from build123d import *

# Parameters (mm, degrees)
SKETCH1_W           = 80
SKETCH1_H           = 100
SKETCH1_R           = 2.1
SKETCH1_R_2         = 2.5
BOSS_EXTRUDE1_DEPTH = 3


with BuildPart() as part:
    # Sketch1 → Boss-Extrude1 (new body)
    with BuildSketch(Plane(origin=(0, 0, 0), x_dir=(1, 0, 0), z_dir=(0, 1, 0))):
        Rectangle(SKETCH1_W, SKETCH1_H)
        with Locations(Location((24.5, 42, 0), (0, 0, 90))):
            Circle(SKETCH1_R, mode=Mode.SUBTRACT)
        with Locations(Location((-24.5, 42, 0), (0, 0, 270))):
            Circle(SKETCH1_R, mode=Mode.SUBTRACT)
        with Locations(Location((24.5, -40, 0), (0, 0, 270))):
            Circle(SKETCH1_R, mode=Mode.SUBTRACT)
        with Locations(Location((-24.5, -40, 0), (0, 0, 270))):
            Circle(SKETCH1_R, mode=Mode.SUBTRACT)
        with Locations(Location((10, -10, 0), (0, 0, 270))):
            Circle(SKETCH1_R, mode=Mode.SUBTRACT)
        with Locations(Location((-10, -10, 0), (0, 0, 270))):
            Circle(SKETCH1_R, mode=Mode.SUBTRACT)
        with Locations(Location((0, -27, 0), (0, 0, 270))):
            Circle(SKETCH1_R_2, mode=Mode.SUBTRACT)
    extrude(amount=BOSS_EXTRUDE1_DEPTH)


solid = part.part
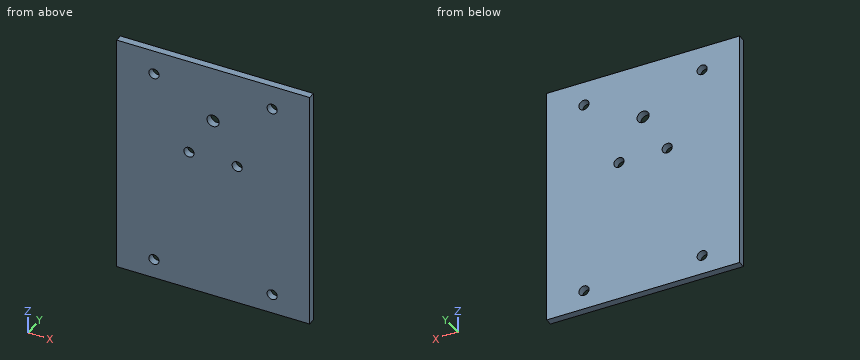
Source: CAD feature listing. Evaluate the final solid. Frame: model axes, mm. Give positions to 0.01 mm unless a question says otherwise; leave off trailing zeros. Write each loop counter-clockwise with the first axis right and the second up, starting at its lowest first coordinate (ties: lowest second). Pieces come first, ordered by that corner, then holes. Notation, with made-up numbers: M 53,67 L 67,67 A16 cw 67,73 Z; hole C 40,-13 d10. An arc over 180 degrees is marked long. Answer as a JSON object with one key per item and string values.
Q1. Cut plane C-C, the plane x = 24.5. Return the cut outline in (y, z).
Geometry check:
{"outline": "M 0,-50 L 3,-50 L 3,-44.1 L 0,-44.1 Z; M 0,-39.9 L 3,-39.9 L 3,37.9 L 0,37.9 Z; M 0,42.1 L 3,42.1 L 3,50 L 0,50 Z"}
Q2. Cut plane B-B, the plane x = 0. Return the cut outline in (y, z), then the cut area to 3 significant figures.
Geometry check:
{"outline": "M 0,-50 L 3,-50 L 3,24.5 L 0,24.5 Z; M 0,29.5 L 3,29.5 L 3,50 L 0,50 Z", "area": "285 mm^2"}
Q3. Cut plane A-A, the plane z = 27. Return the cut outline in (x, y).
Geometry check:
{"outline": "M -40,0 L -2.5,0 L -2.5,3 L -40,3 Z; M 2.5,0 L 40,0 L 40,3 L 2.5,3 Z"}
Q4. Ray query, line 1 along X through (y, z) = (1.4, 40); line 2 along X through (y, z) = (2.1, 10); line 3 along X through (y, z) = (0.75, 27). Return the intervals inside material, ascending.
Geometry check:
{"line 1": "x = -40 to -26.6, -22.4 to 22.4, 26.6 to 40", "line 2": "x = -40 to -12.1, -7.9 to 7.9, 12.1 to 40", "line 3": "x = -40 to -2.5, 2.5 to 40"}
Q5. Cut plane D-D, the plane z = 10. Return the cut outline in (x, y), then the cut area to 3 significant figures.
Geometry check:
{"outline": "M -40,0 L -12.1,0 L -12.1,3 L -40,3 Z; M -7.9,0 L 7.9,0 L 7.9,3 L -7.9,3 Z; M 12.1,0 L 40,0 L 40,3 L 12.1,3 Z", "area": "215 mm^2"}
Q6. Contact query for flat-ended pins moving along their axis: P1, Ø2.5, axis at x = 24.5, z = 40, coming from the +Y side; P2, Ø5.5, axis at x = 24.5, z = -42, coming from the -Y side. Output: stop coordinate, or through.
Geometry check:
{"P1": "passes through", "P2": "stops at y = 0"}
